```python
from build123d import *

# Parameters (mm, degrees)
F1_DEPTH = 25


with BuildPart() as f1:
    # F0 (on Top) → F1 (new body)
    with BuildSketch(Plane.XY):
        Polygon((10.229582, -0.854153), (4.12538, -0.854153), (-4.248491, -0.854153), (-10.229582, -0.854153), (-10.229582, -69.679364), (10.229582, -69.679364), align=None)
        Polygon((13.568254, 11.691391), (13.568254, 18.818088), (-13.691364, 18.818088), (-13.691364, 11.691391), (-4.248491, 11.691391), (-4.248491, -0.854153), (4.12538, -0.854153), (4.12538, 11.691391), align=None)
    extrude(amount=F1_DEPTH)


solid = f1.part
```
Design review of the part built by this model. Coordinates are the model's own, in mm. A direction names the side the tool comes from. Give positions to 0.01 mm unless a question says otherwise; leave off trailing zeros. Order: outer loops, then holes, each group sorted by start corner. A loop starts at its lowest first (then second) coordinate and runs counter-clockwise, first axis right, second up. Notation, with made-up numbers: (37.5, 67.5) -> (79.5, 67.5) arc R19 ccw to (79.5, 103.5) -> close; hole circle Ø2 at (61, -24.75). An arc over 180 degrees is marked (long way). Write each question's results on one line, items separated by ' | '. Start each with the question number.
Q1. For pin 1 (12 mm diameter, centred on y = -33.5, z = 15.5, fed in from -X); pin 2 (4 mm diameter, centred on y = 4.5, z = 14.5, fed in from -X); pin 3 (4 mm diameter, centred on y = 3, z = 17, fed in from +X), all flat-tipped, find the tip position at first contact; note any pin that passes through.
Q2. Machinability: for faces 1 (the flat face through (-4.248, 6, 12)), 2 (the flat face through (0, -69.679, 12)), 3 (the flat face through (-10.23, -35, 12)), 4 (the flat face through (10.23, -36, 12)), 5 (the flat face through (9, 11.691, 12)), which of the approach directions +Z, -Z, +X, -X, +Y, -Y give a long, thin tool a straight path to every point of the face, cutting with its end or side? Answer none if there is none.
Q3. Wall thickness on L1, parallel to Y at x = -7.75, z = 16.75; L2, parallel to X at y = -50.5, z = 12.25; L3, parallel to Y at x = 10.75, z = 17: over which ranges is each line inside the solid? List them lowest first. Write a range as from..to.
Q4. Add section D-D on y = 2.5. Give the boundary of the cut face in (x, z), and give its area (3 significant figures).
Q5. Add section C-C on y = -57.5. Give the boundary of the cut face in (x, z).
Q6. Add section B-B on z = 23. Give the boundary of the cut face in (x, y).
Q7. Mouldability with a two-part tool opening along Y and no side actions: class faces 6 (the flat face through (0, 18.818, 12)), 7 (the flat face through (-9, 11.691, 12)), 8 (the flat face through (0, -25, 25)) as +Y half, -Y half, draft (parallel to the pull), parting line (faces both ways), or undercut.
Q8. Add section A-A on x = -8. Give the boundary of the cut face in (y, z).
Found:
1) pin 1: stops at x = -10.23 | pin 2: stops at x = -4.25 | pin 3: stops at x = 4.13
2) face 1: +Z, -Z, -X | face 2: +Z, -Z, +X, -X, -Y | face 3: +Z, -Z, -X, -Y | face 4: +Z, -Z, +X, -Y | face 5: +Z, -Z, +X
3) L1: y = -69.68..-0.85, 11.69..18.82 | L2: x = -10.23..10.23 | L3: y = 11.69..18.82
4) outline: (-4.25, 0) -> (4.13, 0) -> (4.13, 25) -> (-4.25, 25) -> close | area: 209 mm2
5) outline: (-10.23, 0) -> (10.23, 0) -> (10.23, 25) -> (-10.23, 25) -> close
6) outline: (-13.69, 11.69) -> (-4.25, 11.69) -> (-4.25, -0.85) -> (-10.23, -0.85) -> (-10.23, -69.68) -> (10.23, -69.68) -> (10.23, -0.85) -> (4.13, -0.85) -> (4.13, 11.69) -> (13.57, 11.69) -> (13.57, 18.82) -> (-13.69, 18.82) -> close
7) face 6: +Y half | face 7: undercut | face 8: draft
8) outline: (-69.68, 0) -> (-0.85, 0) -> (-0.85, 25) -> (-69.68, 25) -> close; (11.69, 0) -> (18.82, 0) -> (18.82, 25) -> (11.69, 25) -> close
